Part model, mm, in its own coordinate system. A direction names the side the tool comes from. Coordinates: 2 decimals unless noted, no trailing zeros. Loops run counter-clockwise (first coordinate to the right, second up) from the corner with the lowest first, then second, coordinate; pieces in that order, holes last.
```python
from build123d import *

# Parameters (mm, degrees)
SKETCH1_R           = 15.6
BOSS_EXTRUDE1_DEPTH = 2
BOSS_EXTRUDE3_DEPTH = 122.8
SKETCH11_R          = 14.65
BOSS_EXTRUDE4_DEPTH = 9
CUT_EXTRUDE1_DEPTH  = 1.5
CUT_EXTRUDE2_DEPTH  = 1.5


with BuildPart() as part:
    # Sketch1 → Boss-Extrude1 (new body)
    with BuildSketch(Plane.XY):
        Circle(SKETCH1_R)
    extrude(amount=BOSS_EXTRUDE1_DEPTH)

    # Sketch5 → Boss-Extrude3 (add)
    with BuildSketch(Plane(origin=(0, 0, -122.8), x_dir=(-1, 0, 0), z_dir=(0, 0, -1))):
        Polygon((0.75, 0.75), (13.7, 0.75), (13.7, -0.75), (0.75, -0.75), (0.75, -13.886326313), (-0.75, -13.886326313), (-0.75, -0.75), (-13.7, -0.75), (-13.7, 0.75), (-0.75, 0.75), (-0.75, 13.886326313), (0.75, 13.886326313), align=None)
    extrude(amount=-BOSS_EXTRUDE3_DEPTH)

    # Sketch11 → Boss-Extrude4 (add)
    with BuildSketch(Plane(origin=(0, 0, -122.8), x_dir=(-1, 0, 0), z_dir=(0, 0, -1))):
        Circle(SKETCH11_R)
    extrude(amount=BOSS_EXTRUDE4_DEPTH)

    # Sketch12 → Cut-Extrude1 (cut)
    with BuildSketch(Plane.ZY.offset(0.75)):
        with BuildLine():
            Line((0, 8.228019132), (-15, 8.228019132))
            add(Edge.make_bspline(
                [(-15, 8.228019132), (-24.489612622, 8.228019132), (-24.489612622, 13.886326313), (-35, 13.886326313)],
                knots=[0, 0, 0, 0, 1, 1, 1, 1], degree=3))
            Line((-35, 13.886326313), (-35, 19.520904109))
            Line((-35, 19.520904109), (0, 19.520904109))
            Line((0, 19.520904109), (0, 8.228019132))
        make_face()
        with BuildLine():
            Line((0, -19.520904109), (0, -8.228019132))
            Line((0, -8.228019132), (-15, -8.228019132))
            add(Edge.make_bspline(
                [(-15, -8.228019132), (-24.489612622, -8.228019132), (-24.489612622, -13.886326313), (-35, -13.886326313)],
                knots=[0, 0, 0, 0, 1, 1, 1, 1], degree=3))
            Line((-35, -13.886326313), (-35, -19.520904109))
            Line((-35, -19.520904109), (0, -19.520904109))
        make_face()
    extrude(amount=-CUT_EXTRUDE1_DEPTH, mode=Mode.SUBTRACT)

    # Sketch13 → Cut-Extrude2 (cut)
    with BuildSketch(Plane.XZ.offset(0.75)):
        with BuildLine():
            Line((7.75, 0), (7.75, -15))
            add(Edge.make_bspline(
                [(7.75, -15), (7.75, -21.966675068), (13.7, -21.966675068), (13.7, -35)],
                knots=[0, 0, 0, 0, 1, 1, 1, 1], degree=3))
            Line((13.7, -35), (21.110657524, -35))
            Line((21.110657524, -35), (21.110657524, 0))
            Line((21.110657524, 0), (7.75, 0))
        make_face()
        with BuildLine():
            Line((-21.110657524, 0), (-7.75, 0))
            Line((-7.75, 0), (-7.75, -15))
            add(Edge.make_bspline(
                [(-7.75, -15), (-7.75, -21.966675068), (-13.7, -21.966675068), (-13.7, -35)],
                knots=[0, 0, 0, 0, 1, 1, 1, 1], degree=3))
            Line((-13.7, -35), (-21.110657524, -35))
            Line((-21.110657524, -35), (-21.110657524, 0))
        make_face()
    extrude(amount=-CUT_EXTRUDE2_DEPTH, mode=Mode.SUBTRACT)


solid = part.part
```
Q1. Mould opens along Z. For faces 1 (the flat face through (0, 0, -131.8)), 2 (the flat face through (-0.75, -7, -62)), 3 (the cylindrical face through (-13.973, 4.4, -127.237)), 4 (the flat face through (7, 0.75, -62)) say: released by +Z, released by -Z, zero draft, split by the parting line, or undercut.
Q2. Tool access for faces 5 (the flat face through (-3, -3, -122.8)), 6 (the flat face through (7, -0.75, -62)), 7 (the flat face through (-7, -0.75, -62)), 8 (the flat face through (-0.75, 7, -62)): list every direction of +Z, -Z, +X, -X, +Y, -Y with a clear straight run to the whole face (end or side of a thin tool).
Q3. Saw through at A-A (z = -8). List the corners of the cut face in (x, y), plus the area to 3 significant figures.
Q4. Saw through at B-B (x = 6). List the corners of the cut face in (y, z), plus the area to 3 significant figures.
Q5. Drop flat-ended pins along their axis: P1, Ø3, axis at x = -4, z = -94, coming from the +Y side; P2, Ø1.2, axis at x = 0, z = -6, coming from the -Y side; P3, Ø12, axis at x = 5.5, z = -47, coming from the -Y side. Give the stop position or say it passes through.
Q6. Probe line 1 (Z direction, x = 3.5, y = -10.5); line 2 (X direction, y = 1, z = -113.5). List the from-to ranges inside material, lowest first.
Checked values:
1. face 1: released by -Z
1. face 2: undercut
1. face 3: zero draft
1. face 4: undercut
2. face 5: none
2. face 6: +X, -Y
2. face 7: -X, -Y
2. face 8: -X, +Y
3. outline: (-7.75, -0.75) - (-0.75, -0.75) - (-0.75, -8.23) - (0.75, -8.23) - (0.75, -0.75) - (7.75, -0.75) - (7.75, 0.75) - (0.75, 0.75) - (0.75, 8.23) - (-0.75, 8.23) - (-0.75, 0.75) - (-7.75, 0.75) - close
3. area: 45.7 mm2
4. outline: (-14.4, 0) - (-0.75, 0) - (-0.75, -122.8) - (-13.36, -122.8) - (-13.36, -131.8) - (13.36, -131.8) - (13.36, -122.8) - (0.75, -122.8) - (0.75, 0) - (14.4, 0) - (14.4, 2) - (-14.4, 2) - close
4. area: 482 mm2
5. P1: stops at y = 0.75
5. P2: stops at y = -8.23
5. P3: stops at y = -13.89
6. line 1: z = -131.8 to -122.8, 0 to 2
6. line 2: x = -0.75 to 0.75
